For this review, take the finished solid that the model builds, in its own axes (mm). A direction names the side the tool comes from. Coordinates: 2 decimals unless noted, no trailing zeros. Loops run counter-clockwise (first coordinate to the right, second up) from the corner with the lowest first, then second, coordinate; pieces in that order, holes last. Notation, with made-up numbers: (-4.5, -3.75) - (48.5, -3.75) arc R25 cw to (48.5, 19.25) - close; hole circle Ø7 at (0.5, 49). An arc over 180 degrees is marked (long way). Answer as a JSON object with one key per item and string values. Group by question number.
Item 1: We need section A-A (y = 0). Give the boundary of the cut face in (x, z), then the cut area to 3 significant figures.
Item 2: Mouldability with a two-part tool opening along X and no side actions: class faces 1 (the flat face through (11, -8, 5)), 2 (the flat face through (7.33, 4.24, 4.93)), 3 (the flat face through (-7.95, -4.24, 4.93)) as released by +X, released by -X, zero draft, split by the parting line, or undercut.
Item 3: Tool access review of faces 4 (the cylindrical face through (27.386, -6.158, 5.575)), 5 (the flat face through (2.75, -7, 5)), 6 (the flat face through (-7.17, 4.26, 4.93)), 7 (the flat face through (8, -16, 5)), 8 (the cylindrical face through (15.032, -0.843, 5.563)): name each direction out of +Z, -Z, +X, -X, +Y, -Y from which nothing blocks a thin tool from reaching the whole face with its end or side.
Item 4: We need section D-D (z = 5). Give the boundary of the cut face in (x, y), then the cut area to 3 significant figures.
Item 5: Clearance check with flat-ended pins moving along their axes: pin 1 (1.5 mm diameter, centred on y = -3, z = 4, fed in from +X); pin 2 (6 mm diameter, centred on y = -13.5, z = 3, fed in from -X); pin 3 (2.5 mm diameter, centred on x = -13, y = 0, fed in from +Z); pin 4 (8 mm diameter, centred on x = 7, y = -16.5, fed in from -Z). State where each tip first meets the part, or that it passes through.
Item 6: We need section C-C (z = 2.75). Give the boundary of the cut face in (x, y).
Item 7: We need section B-B (x = 0). Give the boundary of the cut face in (y, z), then the cut area to 3 significant figures.
Item 8: To check wall thickness, follow line 1 (Y direction, x = 13, z = 5); line 2 (Y direction, x = 26, z = 3); line 3 (X direction, y = -6.85, z = 5). State the ranges of each line that lie inside material, in increasing order.
from build123d import *

# Parameters (mm, degrees)
ESQUISSE1_R             = 2.8
ESQUISSE1_W             = 2.75
ESQUISSE1_H             = 8
BOSS_EXTRU_1_DEPTH      = 10
ENL_V_MAT_EXTRU_1_REACH = 17
ESQUISSE2_R             = 1.5
ESQUISSE4_R             = 2.2
ENL_V_MAT_EXTRU_2_DEPTH = 9


with BuildPart() as part:
    # Esquisse1 → Boss.-Extru.1 (new body)
    with BuildSketch(Plane.XY):
        with BuildLine():
            Line((1.5, 5), (-1.5, 5))
            Line((-1.5, 5), (-13, 3.5))
            ThreePointArc((-13, 3.5), (-16.5, 0), (-13, -3.5))
            Line((-13, -3.5), (-2.75, -5))
            Line((-2.75, -5), (2.75, -5))
            Line((2.75, -5), (13, -3.5))
            ThreePointArc((13, -3.5), (16.5, 0), (13, 3.5))
            Line((13, 3.5), (1.5, 5))
        make_face()
        Circle(ESQUISSE1_R, mode=Mode.SUBTRACT)
        Polygon((2.75, -5), (-2.75, -5), (-2.75, -16), (0, -16), (0, -8), (2.75, -8), align=None)
        with Locations((1.375, -12)):
            Rectangle(ESQUISSE1_W, ESQUISSE1_H)
        with BuildLine():
            Line((19.65571123, -8), (2.75, -8))
            Line((2.75, -8), (2.75, -16))
            Line((2.75, -16), (19.65571123, -16))
            ThreePointArc((19.65571123, -16), (18.5, -12), (19.65571123, -8))
        make_face()
        with BuildLine():
            ThreePointArc((33.5, -12), (28.081806214, -4.794718403), (19.65571123, -8))
            Line((19.65571123, -8), (21.6, -8))
            Line((21.6, -8), (21.6, -12))
            Line((21.6, -12), (21.6, -16))
            Line((21.6, -16), (19.65571123, -16))
            ThreePointArc((19.65571123, -16), (28.081806214, -19.205281597), (33.5, -12))
        make_face()
        with BuildLine():
            ThreePointArc((30.4, -12), (26, -16.4), (21.6, -12))
            ThreePointArc((21.6, -12), (26, -7.6), (30.4, -12))
        make_face(mode=Mode.SUBTRACT)
        with BuildLine():
            Line((21.6, -8), (19.65571123, -8))
            ThreePointArc((19.65571123, -8), (18.5, -12), (19.65571123, -16))
            Line((19.65571123, -16), (21.6, -16))
            Line((21.6, -16), (21.6, -12))
            Line((21.6, -12), (21.6, -8))
        make_face()
    extrude(amount=BOSS_EXTRU_1_DEPTH)

    # Esquisse2 → Enlèv. mat.-Extru.1 (cut, up to next)
    with BuildSketch(Plane(origin=(0, -4.5, 0), x_dir=(1, 0, 0), z_dir=(0, 1, 0)), mode=Mode.PRIVATE) as enl_v_mat_extru_1_sk1:
        with Locations((26, -5)):
            Circle(ESQUISSE2_R)
    enl_v_mat_extru_1_tool1 = extrude(enl_v_mat_extru_1_sk1.sketch, amount=-ENL_V_MAT_EXTRU_1_REACH, mode=Mode.PRIVATE) & part.part
    add(enl_v_mat_extru_1_tool1.solids().sort_by_distance((26, -4.5, 5))[0], mode=Mode.SUBTRACT)

    # Esquisse4 → Enlèv. mat.-Extru.2 (cut)
    with BuildSketch(Plane.XY.offset(10)):
        with Locations((-13, 0)):
            Circle(ESQUISSE4_R)
        with Locations((13, 0)):
            Circle(ESQUISSE4_R)
    extrude(amount=-ENL_V_MAT_EXTRU_2_DEPTH, mode=Mode.SUBTRACT)


solid = part.part
Check sheet entries:
{
 "1": {"outline": "(-16.5, 0) - (-2.8, 0) - (-2.8, 10) - (-10.8, 10) - (-10.8, 1) - (-15.2, 1) - (-15.2, 10) - (-16.5, 10) - close; (2.8, 0) - (16.5, 0) - (16.5, 10) - (15.2, 10) - (15.2, 1) - (10.8, 1) - (10.8, 10) - (2.8, 10) - close", "area": "195 mm2"},
 "2": {"face 1": "undercut", "face 2": "released by +X", "face 3": "released by -X"},
 "3": {"face 4": "+Y", "face 5": "+Z, -Z", "face 6": "+Z, -Z, -X, +Y", "face 7": "+Z, -Z, -X, -Y", "face 8": "+Z"},
 "4": {"outline": "(-13, -3.5) - (-2.75, -5) - (-2.75, -16) - (19.66, -16) arc R7.5 ccw (long way) to (27.5, -4.65) - (27.5, -7.86) arc R4.4 cw (long way) to (24.5, -7.86) - (24.5, -4.65) arc R7.5 ccw to (19.66, -8) - (2.75, -8) - (2.75, -5) - (13, -3.5) arc R3.5 ccw to (13, 3.5) - (1.5, 5) - (-1.5, 5) - (-13, 3.5) arc R3.5 ccw to start; hole circle Ø4.4 at (-13, 0); hole circle Ø5.6 at (0, 0); hole circle Ø4.4 at (13, 0)", "area": "507 mm2"},
 "5": {"pin 1": "stops at x = 15.68", "pin 2": "stops at x = -2.75", "pin 3": "stops at z = 1", "pin 4": "stops at z = 0"},
 "6": {"outline": "(-13, -3.5) - (-2.75, -5) - (-2.75, -16) - (19.66, -16) arc R7.5 ccw (long way) to (19.66, -8) - (2.75, -8) - (2.75, -5) - (13, -3.5) arc R3.5 ccw to (13, 3.5) - (1.5, 5) - (-1.5, 5) - (-13, 3.5) arc R3.5 ccw to start; hole circle Ø4.4 at (-13, 0); hole circle Ø5.6 at (0, 0); hole circle Ø4.4 at (13, 0); hole circle Ø8.8 at (26, -12)"},
 "7": {"outline": "(-16, 0) - (-2.8, 0) - (-2.8, 10) - (-16, 10) - close; (2.8, 0) - (5, 0) - (5, 10) - (2.8, 10) - close", "area": "154 mm2"},
 "8": {"line 1": "y = -16 to -8, -3.5 to -2.2, 2.2 to 3.5", "line 2": "y = -19.5 to -16.4, -7.6 to -4.5", "line 3": "x = -2.75 to 2.75, 20.55 to 24.5, 27.5 to 31.45"}
}
